Could you check a few things on this model? Use its own coordinates, in mm. A direction names the side the tool comes from. Coordinates: 2 decimals unless noted, no trailing zeros. Loops run counter-clockwise (first coordinate to the right, second up) from the corner with the lowest first, then second, coordinate; pieces in that order, holes last. Notation, with made-up numbers: (8, 80.25) - (53, 80.25) arc R36 cw to (53, 118.25) - close; hole circle Ø7 at (-38, 7.5). An arc over 180 degrees is marked (long way). Put each result on its own line as item: value. Start each with the question number.
```python
from build123d import *

# Parameters (mm, degrees)
SKETCH1_R           = 3
BOSS_EXTRUDE1_DEPTH = 1.75
SKETCH2_R           = 1.5
BOSS_EXTRUDE2_DEPTH = 10
CHAMFER1_SIZE       = 1.7
CHAMFER2_SIZE       = 0.25


with BuildPart() as part:
    # Sketch1 → Boss-Extrude1 (new body)
    with BuildSketch(Plane(origin=(0, 0, 0), x_dir=(1, 0, 0), z_dir=(0, 1, 0))):
        with Locations(Location((0, 0, 0), (0, 0, 270))):
            Circle(SKETCH1_R)
    extrude(amount=BOSS_EXTRUDE1_DEPTH)

    # Sketch2 → Boss-Extrude2 (add)
    with BuildSketch(Plane(origin=(0, 1.75, 0), x_dir=(1, 0, 0), z_dir=(0, 1, 0))):
        with Locations(Location((0, 0, 0), (0, 0, 270))):
            Circle(SKETCH2_R)
    extrude(amount=BOSS_EXTRUDE2_DEPTH)

    # Chamfer1
    # the kernel refuses this chamfer: 1.7 mm, written as the material it takes off along each edge
    with BuildSketch(Plane(origin=(0, 1.75, 0), x_dir=(0, 0, 1), z_dir=(-1, 0, 0))) as chamfer1_piece_1_section:
        Polygon((3, -CHAMFER1_SIZE), (3 - CHAMFER1_SIZE, 0), (3, 0), align=None)
    chamfer1_piece_1 = revolve(axis=Axis((0, 1.75, 0), (0, 1, 0)), mode=Mode.PRIVATE)
    chamfer1_piece_1 = chamfer1_piece_1 - Plane(origin=(0, 0.796367942, 0), x_dir=(0, 0, 1), z_dir=(0, -1, 0)) * Cylinder(1.5, 12, mode=Mode.PRIVATE)
    add(chamfer1_piece_1, mode=Mode.SUBTRACT)

    # Chamfer2
    chamfer2_edges = [part.edges().sort_by_distance(p)[0] for p in [
        (0, 11.75, -1.5),
    ]]
    chamfer(chamfer2_edges, length=CHAMFER2_SIZE)


solid = part.part
```
(1) I want a section at B-B on z = 0. List the corners of the cut face in (x, y) for me.
(2) I want a section at A-A on x = 0. List the corners of the cut face in (y, z) for me.
(3) For pin 1 Ø3 at (y, z) = (9.5, 1.5) entering from +X; pin 2 Ø3 at (x, y) = (-1.5, 7.5) entering from -Z; pin 3 Ø1 at (x, z) = (-1, -2) entering from +Y, each with a flat end and sliding along its axis, tell me the tip position at first contact or that it passes through.
(4) I need wall thicknesses on L1, parallel to X at y = 2.5, z = 0.1; L2, parallel to Z at x = -1.1, y = 2.25. Which ranges of each line are inside material? Lowest first, please. Write a range as [from, to].
(5) I want a section at C-C on y = 5.25. List the corners of the cut face in (x, z) for me.
(6) Which directions (+Z, -Z, +X, -X, +Y, -Y) give clear straight access to the entire face, cutting with the end or side of a thin tool? Please do faces 1 (the flat face through (0, 11.75, 0)), 2 (the cylindrical face through (-0.07, 6.46, -1.5)).
Answer sheet:
1. outline: (-3, 0) - (3, 0) - (3, 0.05) - (1.5, 1.55) - (1.5, 11.5) - (1.25, 11.75) - (-1.25, 11.75) - (-1.5, 11.5) - (-1.5, 1.55) - (-3, 0.05) - close
2. outline: (0, -3) - (0.05, -3) - (1.55, -1.5) - (11.5, -1.5) - (11.75, -1.25) - (11.75, 1.25) - (11.5, 1.5) - (1.55, 1.5) - (0.05, 3) - (0, 3) - close
3. pin 1: stops at x = 1.5
3. pin 2: stops at z = -1.5
3. pin 3: stops at y = 1.31
4. L1: x = [-1.5, 1.5]
4. L2: z = [-1.02, 1.02]
5. outline: circle Ø3 at (0, 0)
6. face 1: +Z, -Z, +X, -X, +Y
6. face 2: +Y
